Model file for the job. Use its own axes, mm. Face numbers are marked on the shaded views. Coordinates: 2 decimals unless noted, no trailing zeros. Loops run counter-clockwise (first coordinate to the right, second up) from the corner with the lowest first, then second, coordinate; pieces in that order, holes last. Notation, with made-up numbers: (-39, 40.25) -> (-20, 40.25) arc R19 cw to (-20, 77.25) -> close; hole circle Ø7 at (-9.75, 46). An arc over 180 degrees is marked (long way). Use one line per item in the form item = value.
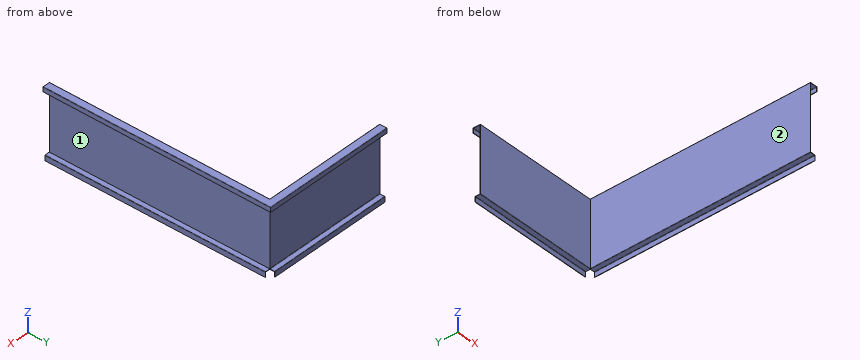
```python
from build123d import *

# Parameters (mm, degrees)
F3_W         = 27
F3_H         = 27
F4_DEPTH     = 30
F5_T1_DEPTH  = 666
F5_T3_DEPTH  = 702
F5_T5_DEPTH  = 1176
F5_T7_DEPTH  = 1212
F5_T13_DEPTH = 1181
F5_T17_DEPTH = 671
F5_T20_DEPTH = 669
F5_T22_DEPTH = 676
F5_T24_DEPTH = 714
F5_T26_DEPTH = 1224
F5_T28_DEPTH = 1179
F5_T30_DEPTH = 1186
F5_T36_DEPTH = 674
F5_T40_DEPTH = 1184
F5_T47_DEPTH = 674
F5_T51_DEPTH = 1184


# Not quite as in the source:
# - a fillet or chamfer that OpenCascade refuses, or shapes differently, is made with other operations: its cross-section is extruded or revolved along the edge and cut away or added


with BuildPart() as f2:
    # F2: sweep along a path in F1
    with BuildLine(Plane.XY) as f2_path:
        Line((0, 0), (0, 1174))
        Line((0, 1174), (-664, 1174))
    # F0 (on Front) → F2 (sweep)
    with BuildSketch(Plane.XZ):
        Polygon((38, -2), (38, -25), (40, -25), (40, 0), (0, 0), (0, -350), (27, -350), (27, -376), (29, -376), (29, -348), (2, -348), (2, -2), align=None)
    sweep(path=f2_path.line, transition=Transition.RIGHT)

    # F3 (on face) → F4 (cut)
    with BuildSketch(Plane.XY.offset(-348)):
        with Locations((15.5, 1189.5)):
            Rectangle(F3_W, F3_H)
    extrude(amount=-F4_DEPTH, mode=Mode.SUBTRACT)

    # F5: fillet of radius 2 on 15 edges, made by hand

    # F5_s2 → F5_t1 (join)
    with BuildSketch(Plane.YZ.offset(-664)):
        with BuildLine():
            ThreePointArc((1199, -350), (1200.4142135624, -350.5857864376), (1201, -352))
            Line((1201, -352), (1201, -350))
            Line((1201, -350), (1199, -350))
        make_face()
        with BuildLine():
            ThreePointArc((1176, -346), (1176.5857864376, -347.4142135624), (1178, -348))
            Line((1178, -348), (1176, -348))
            Line((1176, -348), (1176, -346))
        make_face()
        with BuildLine():
            ThreePointArc((1178, -2), (1176.5857864376, -2.5857864376), (1176, -4))
            Line((1176, -4), (1176, -2))
            Line((1176, -2), (1178, -2))
        make_face()
    extrude(amount=F5_T1_DEPTH)

    # F5_s4 → F5_t3 (join)
    with BuildSketch(Plane.YZ.offset(-664)):
        with BuildLine():
            ThreePointArc((1210, -2), (1211.4142135624, -2.5857864376), (1212, -4))
            Line((1212, -4), (1212, -2))
            Line((1212, -2), (1210, -2))
        make_face()
    extrude(amount=F5_T3_DEPTH)

    # F5_s6 → F5_t5 (join)
    with BuildSketch(Plane.XZ.offset(-1176)):
        with BuildLine():
            ThreePointArc((25, -350), (26.4142135624, -350.5857864376), (27, -352))
            Line((27, -352), (27, -350))
            Line((27, -350), (25, -350))
        make_face()
        with BuildLine():
            ThreePointArc((4, -2), (2.5857864376, -2.5857864376), (2, -4))
            Line((2, -4), (2, -2))
            Line((2, -2), (4, -2))
        make_face()
    extrude(amount=F5_T5_DEPTH)

    # F5_s8 → F5_t7 (join)
    with BuildSketch(Plane.XZ.offset(-1212)):
        with BuildLine():
            ThreePointArc((38, -4), (37.4142135624, -2.5857864376), (36, -2))
            Line((36, -2), (38, -2))
            Line((38, -2), (38, -4))
        make_face()
    extrude(amount=F5_T7_DEPTH)


with BuildPart() as f5_tool11:
    # F5_s12 → F5_t13 (new body)
    with BuildSketch(Plane.XZ):
        with BuildLine():
            ThreePointArc((4, -2), (2.5857864376, -2.5857864376), (2, -4))
            Line((2, -4), (2, -2))
            Line((2, -2), (4, -2))
        make_face()
    extrude(amount=-F5_T13_DEPTH)

    split(bisect_by=Plane.XZ.offset(-1176), keep=Keep.BOTTOM)


with BuildPart() as f5_tool15:
    # F5_s16 → F5_t17 (new body)
    with BuildSketch(Plane.YZ.offset(7)):
        with BuildLine():
            ThreePointArc((1178, -2), (1176.5857864376, -2.5857864376), (1176, -4))
            Line((1176, -4), (1176, -2))
            Line((1176, -2), (1178, -2))
        make_face()
    extrude(amount=-F5_T17_DEPTH)

    split(bisect_by=Plane.YZ.offset(2), keep=Keep.TOP)


with BuildPart() as f5_tool11_1:
    add(f5_tool11.part)

    # F5_t19: intersect F5_tool15
    add(f5_tool15.part, mode=Mode.INTERSECT)


with BuildPart() as f2_1:
    add(f2.part)

    # F5_t9: union F5_tool11
    add(f5_tool11_1.part)

    # F5_s21 → F5_t20 (cut)
    with BuildSketch(Plane.YZ.offset(-669)):
        with BuildLine():
            ThreePointArc((1174, -348), (1174.5857864376, -349.4142135624), (1176, -350))
            Line((1176, -350), (1174, -350))
            Line((1174, -350), (1174, -348))
        make_face()
        with BuildLine():
            ThreePointArc((1174, -2), (1174.5857864376, -0.5857864376), (1176, 0))
            Line((1176, 0), (1174, 0))
            Line((1174, 0), (1174, -2))
        make_face()
    extrude(amount=F5_T20_DEPTH, mode=Mode.SUBTRACT)

    # F5_s23 → F5_t22 (cut)
    with BuildSketch(Plane.YZ.offset(-669)):
        with BuildLine():
            ThreePointArc((1201, -348), (1202.4142135624, -348.5857864376), (1203, -350))
            Line((1203, -350), (1203, -348))
            Line((1203, -348), (1201, -348))
        make_face()
    extrude(amount=F5_T22_DEPTH, mode=Mode.SUBTRACT)

    # F5_s25 → F5_t24 (cut)
    with BuildSketch(Plane.YZ.offset(-669)):
        with BuildLine():
            ThreePointArc((1214, -2), (1213.4142135624, -0.5857864376), (1212, 0))
            Line((1212, 0), (1214, 0))
            Line((1214, 0), (1214, -2))
        make_face()
    extrude(amount=F5_T24_DEPTH, mode=Mode.SUBTRACT)

    # F5_s27 → F5_t26 (cut)
    with BuildSketch(Plane.XZ.offset(-1219)):
        with BuildLine():
            ThreePointArc((38, 0), (39.4142135624, -0.5857864376), (40, -2))
            Line((40, -2), (40, 0))
            Line((40, 0), (38, 0))
        make_face()
    extrude(amount=F5_T26_DEPTH, mode=Mode.SUBTRACT)

    # F5_s29 → F5_t28 (cut)
    with BuildSketch(Plane.XZ.offset(-1174)):
        with BuildLine():
            ThreePointArc((0, -2), (0.5857864376, -0.5857864376), (2, 0))
            Line((2, 0), (0, 0))
            Line((0, 0), (0, -2))
        make_face()
        with BuildLine():
            ThreePointArc((2, -350), (0.5857864376, -349.4142135624), (0, -348))
            Line((0, -348), (0, -350))
            Line((0, -350), (2, -350))
        make_face()
    extrude(amount=F5_T28_DEPTH, mode=Mode.SUBTRACT)

    # F5_s31 → F5_t30 (cut)
    with BuildSketch(Plane.XZ.offset(-1181)):
        with BuildLine():
            ThreePointArc((27, -348), (28.4142135624, -348.5857864376), (29, -350))
            Line((29, -350), (29, -348))
            Line((29, -348), (27, -348))
        make_face()
    extrude(amount=F5_T30_DEPTH, mode=Mode.SUBTRACT)


with BuildPart() as f5_tool34:
    # F5_s35 → F5_t36 (new body)
    with BuildSketch(Plane.YZ.offset(5)):
        with BuildLine():
            ThreePointArc((1174, -348), (1174.5857864376, -349.4142135624), (1176, -350))
            Line((1176, -350), (1174, -350))
            Line((1174, -350), (1174, -348))
        make_face()
    extrude(amount=-F5_T36_DEPTH)

    split(bisect_by=Plane.YZ, keep=Keep.TOP)


with BuildPart() as f5_tool38:
    # F5_s39 → F5_t40 (new body)
    with BuildSketch(Plane.XZ.offset(5)):
        with BuildLine():
            ThreePointArc((2, -350), (0.5857864376, -349.4142135624), (0, -348))
            Line((0, -348), (0, -350))
            Line((0, -350), (2, -350))
        make_face()
    extrude(amount=-F5_T40_DEPTH)

    split(bisect_by=Plane.XZ.offset(-1174), keep=Keep.BOTTOM)


with BuildPart() as f5_tool34_1:
    add(f5_tool34.part)

    # F5_t42: intersect F5_tool38
    add(f5_tool38.part, mode=Mode.INTERSECT)


with BuildPart() as f2_2:
    add(f2_1.part)

    # F5_t32: cut F5_tool34
    add(f5_tool34_1.part, mode=Mode.SUBTRACT)


with BuildPart() as f5_tool45:
    # F5_s46 → F5_t47 (new body)
    with BuildSketch(Plane.YZ.offset(5)):
        with BuildLine():
            ThreePointArc((1174, -2), (1174.5857864376, -0.5857864376), (1176, 0))
            Line((1176, 0), (1174, 0))
            Line((1174, 0), (1174, -2))
        make_face()
    extrude(amount=-F5_T47_DEPTH)

    split(bisect_by=Plane.YZ, keep=Keep.TOP)


with BuildPart() as f5_tool49:
    # F5_s50 → F5_t51 (new body)
    with BuildSketch(Plane.XZ.offset(5)):
        with BuildLine():
            ThreePointArc((0, -2), (0.5857864376, -0.5857864376), (2, 0))
            Line((2, 0), (0, 0))
            Line((0, 0), (0, -2))
        make_face()
    extrude(amount=-F5_T51_DEPTH)

    split(bisect_by=Plane.XZ.offset(-1174), keep=Keep.BOTTOM)


with BuildPart() as f5_tool45_1:
    add(f5_tool45.part)

    # F5_t53: intersect F5_tool49
    add(f5_tool49.part, mode=Mode.INTERSECT)


with BuildPart() as f2_3:
    add(f2_2.part)

    # F5_t43: cut F5_tool45
    add(f5_tool45_1.part, mode=Mode.SUBTRACT)


solid = f2_3.part
```
Q1. Band-saw the part on C-C, the plane z = -82.5. Write the cut outline in (x, y), and give its area (3 significant figures).
Result:
outline = (-664, 1174) -> (0, 1174) -> (0, 0) -> (2, 0) -> (2, 1176) -> (-664, 1176) -> close
area = 3,680 mm2
Q2. Mould opens along Z. For the marked faces 1 and 2 say: released by +Z, released by -Z, zero draft, split by the parting line, or undercut.
Result:
face_1 = undercut
face_2 = zero draft
Q3. Band-saw the part on B-B, the plane y = 830. Write the cut outline in (x, z), and give its area (3 significant figures).
Result:
outline = (0, -348) arc R2 ccw to (2, -350) -> (25, -350) arc R2 cw to (27, -352) -> (27, -376) -> (29, -376) -> (29, -350) arc R2 ccw to (27, -348) -> (2, -348) -> (2, -4) arc R2 cw to (4, -2) -> (36, -2) arc R2 cw to (38, -4) -> (38, -25) -> (40, -25) -> (40, -2) arc R2 ccw to (38, 0) -> (2, 0) arc R2 ccw to (0, -2) -> close
area = 927 mm2
Q4. Pin check, flat tips, straight feed: pin 1 Ø3 at (x, z) = (-288, -98.5) entering from -Y; pin 2 Ø17 at (y, z) = (906, -13.5) entering from -X; pin 3 Ø7 at (x, y) = (-448, 1191.5) entering from -Z. Stop position of each tip, or through.
Result:
pin_1 = 1174
pin_2 = 0
pin_3 = -350
Q5. Wall check: line 1 along X through (y, z) = (386, -21); line 2 along Y through (x, z) = (-164, -100); line 3 along X through (y, z) = (740, -207). Give the ranges that are in metal, low to high.
Result:
line_1 = 0 to 2, 38 to 40
line_2 = 1174 to 1176
line_3 = 0 to 2
Q6. Band-saw the part on A-A, the plane x = -29. Write the cut outline in (y, z).
Result:
outline = (1174, -348) arc R2 ccw to (1176, -350) -> (1199, -350) arc R2 cw to (1201, -352) -> (1201, -376) -> (1203, -376) -> (1203, -350) arc R2 ccw to (1201, -348) -> (1178, -348) arc R2 cw to (1176, -346) -> (1176, -4) arc R2 cw to (1178, -2) -> (1210, -2) arc R2 cw to (1212, -4) -> (1212, -25) -> (1214, -25) -> (1214, -2) arc R2 ccw to (1212, 0) -> (1176, 0) arc R2 ccw to (1174, -2) -> close
